Autodesk Inventor part; units mm, degrees
ref_plane "YZ Plane" through (0, 0, 0) normal (1, 0, 0) x (0, 1, 0)
ref_plane "XZ Plane" through (0, 0, 0) normal (0, 1, 0) x (-1, 0, 0)
ref_plane "XY Plane" through (0, 0, 0) normal (0, 0, 1) x (1, 0, 0)
sketch "Sketch1" plane through (0, 0, 0) normal (0, 1, 0) x (-1, 0, 0)
  circle A0 centre (0, 0) radius 16
  dimension "d0" = 32
extrude "Extrusion1" add sketch "Sketch1" along normal blind 19
sketch "Sketch2" plane through (0, 19, 0) normal (0, 1, 0) x (1, 0, 0)
  circle A0 centre (0, 0) radius 3
  dimension "d3" = 6
extrude "Extrusion2" add sketch "Sketch2" along normal blind 2
sketch "Sketch3" plane through (0, 21, 0) normal (0, 1, 0) x (1, 0, 0)
  circle A0 centre (0, 0) radius 1
  dimension "d6" = 2
extrude "Extrusion3" add sketch "Sketch3" along normal blind 9
sketch "Sketch4" plane through (0, 19, 0) normal (0, 1, 0) x (1, 0, 0)
  circle A0 centre (0, 0) radius 12
  line L0 (-12, 0) -> (-11, 0)
  circle A1 centre (11, 0) radius 1
  circle A2 centre (-11, 0) radius 1
  dimension "d9" = 24
extrude "Extrusion4" cut sketch "Sketch4" against normal blind 2 contours A2 | A1
sketch "Sketch5" plane through (0, 0, 0) normal (0, -1, 0) x (1, 0, 0)
  circle A0 centre (-11, 0) radius 1
  circle A1 centre (11, 0) radius 1
  point P0 (0, 0)
extrude "Extrusion5" add sketch "Sketch5" along normal blind 2
properties part number "Motor sensor"
Build history of the part. All positions in model axes, mm. A direction names the side the tool comes from. Coordinates: 2 decimals unless noted, no trailing zeros. Write each loop counter-clockwise with the first axis right and the second up, starting at its lowest first coordinate (ties: lowest second). Pieces come first, ordered by that corner, then holes. Notation, with made-up numbers: (-23, -22) -> (6, -22) arc R5 cw to (6, -13) -> close; hole circle Ø10 at (-1, 67.25). An arc over 180 degrees is marked (long way). Use CSV: the item, a comma, the result in double quotes. Start each with the question number.
Q1. Drill centre lines: probe 1 along Y at (x, z) = (-5, 7); probe 2 along Z at (x, y) = (11, 18.35); probe 3 along Y at (x, z) = (-2.5, -1). Where is each one in solid material? Low to high.
Q2. Cut at B-B, the plane z = 0. List the corners of the cut face in (x, y).
Q3. Cut at D-D, the plane x = -11. List the corners of the cut face in (y, z), then the cut area to 3 significant figures.
Q4. Flat gauge pins, fed straight in: pin 1 Ø1 at (x, z) = (11, 0) entering from +Y; pin 2 Ø1 at (x, z) = (-4, -10) entering from -Y; pin 3 Ø8 at (x, z) = (2.5, 8.5) entering from +Y. Where does each tip first touch, or does it go through?
Q5. 3-axis set-ups, long thin cutter, end or side, ignore diameter. For faces 1 (the cylindrical face through (10.2, -1, 0.6)), 2 (the flat face through (-1, 21, -1)), 3 (the cylindrical face through (3.47, 9.37, 15.62)): which of +Z, -Z, +X, -X, +Y, -Y reach the whole face in a straight line?
Q6. Cut at A-A, the plane x = 0. List the corners of the cut face in (y, z).
Q7. Cut at C-C, the plane y = 20. List the corners of the cut face in (x, z).
Q8. Pull direction X, two halves, no side cores. Call faces 4 (the cylindrical face through (-3, 20, 0)), 5 (the cylindrical face through (-11.8, 18, 0.6)), 6 (the flat face through (11, -2, 0)): released by +X, released by -X, zero draft, split by the parting line, or undercut.
Checked values:
1,probe 1,"y = 0 to 19"
1,probe 2,"z = -11.62 to -1, 1 to 11.62"
1,probe 3,"y = 0 to 21"
2,outline,"(-16, 0) -> (-12, 0) -> (-12, -2) -> (-10, -2) -> (-10, 0) -> (10, 0) -> (10, -2) -> (12, -2) -> (12, 0) -> (16, 0) -> (16, 19) -> (12, 19) -> (12, 17) -> (10, 17) -> (10, 19) -> (3, 19) -> (3, 21) -> (1, 21) -> (1, 30) -> (-1, 30) -> (-1, 21) -> (-3, 21) -> (-3, 19) -> (-10, 19) -> (-10, 17) -> (-12, 17) -> (-12, 19) -> (-16, 19) -> close"
3,outline,"(-2, -1) -> (0, -1) -> (0, -11.62) -> (19, -11.62) -> (19, -1) -> (17, -1) -> (17, 1) -> (19, 1) -> (19, 11.62) -> (0, 11.62) -> (0, 1) -> (-2, 1) -> close"
3,area,"442 mm²"
4,pin 1,"stops at y = 17"
4,pin 2,"stops at y = 0"
4,pin 3,"stops at y = 19"
5,face 1,"-Y"
5,face 2,"+Y"
5,face 3,"+Y, -Y"
6,outline,"(0, -16) -> (19, -16) -> (19, -3) -> (21, -3) -> (21, -1) -> (30, -1) -> (30, 1) -> (21, 1) -> (21, 3) -> (19, 3) -> (19, 16) -> (0, 16) -> close"
7,outline,"circle Ø6 at (0, 0)"
8,face 4,"split by the parting line"
8,face 5,"undercut"
8,face 6,"zero draft"
